Input: part model. Units: mm. Frame: model coordinates. A direction names the side the tool comes from. Give positions to 0.01 mm unless a question says otherwise; leave off trailing zeros. Loops run counter-clockwise (first coordinate to the right, second up) from the corner with the lowest first, then second, coordinate; pieces in that order, holes last. Notation, with made-up numbers: (44.5, 58) -> (52.5, 58) arc R17 cw to (52.5, 69) -> close; hole circle Ø9 at (71.5, 41). An arc over 180 degrees is marked (long way). Answer as a JSON object with one key per item and string values. Group by question number.
```python
from build123d import *

# Parameters (mm, degrees)
BOSS_EXTRUDE1_DEPTH = 6.35
CHAMFER1_SIZE       = 0.79375
CHAMFER2_SIZE       = 1.5875


with BuildPart() as part:
    # Sketch1 → Boss-Extrude1 (new body)
    with BuildSketch(Plane.XY):
        with BuildLine():
            Line((134.621545702, -67.612541882), (134.621545702, -60.810273898))
            ThreePointArc((134.621545702, -60.810273898), (134.621545702, -59.687741882), (133.499013687, -59.687741882))
            Line((133.499013687, -59.687741882), (102.049077718, -59.687741882))
            ThreePointArc((102.049077718, -59.687741882), (100.926545702, -59.687741882), (100.926545702, -60.810273898))
            Line((100.926545702, -60.810273898), (100.926545702, -67.612541882))
            Line((100.926545702, -67.612541882), (95.926545702, -67.612541882))
            Line((95.926545702, -67.612541882), (95.926545702, -60.810273898))
            ThreePointArc((95.926545702, -60.810273898), (95.926545702, -59.687741882), (94.804013687, -59.687741882))
            Line((94.804013687, -59.687741882), (-87.460922281, -59.687741882))
            ThreePointArc((-87.460922281, -59.687741882), (-88.583454296, -59.687741882), (-88.583454296, -60.810273898))
            Line((-88.583454296, -60.810273898), (-88.583454296, -67.612541882))
            Line((-88.583454296, -67.612541882), (-93.583454296, -67.612541882))
            Line((-93.583454296, -67.612541882), (-93.583454296, -60.810273898))
            ThreePointArc((-93.583454296, -60.810273898), (-93.583454296, -59.687741882), (-94.705986312, -59.687741882))
            Line((-94.705986312, -59.687741882), (-126.155922281, -59.687741882))
            ThreePointArc((-126.155922281, -59.687741882), (-127.278454296, -59.687741882), (-127.278454296, -60.810273898))
            Line((-127.278454296, -60.810273898), (-127.278454296, -67.612541882))
            Line((-127.278454296, -67.612541882), (-131.507694323, -67.612541882))
            Line((-131.507694323, -67.612541882), (-131.507694323, -62.385073898))
            ThreePointArc((-131.507694323, -62.385073898), (-131.507694323, -61.262541882), (-132.630226338, -61.262541882))
            Line((-132.630226338, -61.262541882), (-133.628454296, -61.262541882))
            Line((-133.628454296, -61.262541882), (-133.628454296, -60.810273898))
            ThreePointArc((-133.628454296, -60.810273898), (-133.628454296, -59.687741882), (-134.750986312, -59.687741882))
            Line((-134.750986312, -59.687741882), (-139.978454296, -59.687741882))
            Line((-139.978454296, -59.687741882), (-139.978454296, -58.735073898))
            ThreePointArc((-139.978454296, -58.735073898), (-139.978454296, -57.612541882), (-141.100986312, -57.612541882))
            Line((-141.100986312, -57.612541882), (-146.328454296, -57.612541882))
            Line((-146.328454296, -57.612541882), (-146.328454296, -47.612541882))
            Line((-146.328454296, -47.612541882), (-141.100986312, -47.612541882))
            ThreePointArc((-141.100986312, -47.612541882), (-139.978454296, -47.612541882), (-139.978454296, -46.490009867))
            Line((-139.978454296, -46.490009867), (-139.978454296, -38.735073898))
            ThreePointArc((-139.978454296, -38.735073898), (-139.978454296, -37.612541882), (-141.100986312, -37.612541882))
            Line((-141.100986312, -37.612541882), (-146.328454296, -37.612541882))
            Line((-146.328454296, -37.612541882), (-146.328454296, -27.612541882))
            Line((-146.328454296, -27.612541882), (-141.100986312, -27.612541882))
            ThreePointArc((-141.100986312, -27.612541882), (-139.978454296, -27.612541882), (-139.978454296, -26.490009867))
            Line((-139.978454296, -26.490009867), (-139.978454296, -20.787541882))
            Line((-139.978454296, -20.787541882), (-136.575986312, -20.787541882))
            ThreePointArc((-136.575986312, -20.787541882), (-135.453454296, -20.787541882), (-135.453454296, -19.665009867))
            Line((-135.453454296, -19.665009867), (-135.453454296, -17.612541882))
            Line((-135.453454296, -17.612541882), (-125.453454296, -17.612541882))
            Line((-125.453454296, -17.612541882), (-125.453454296, -19.665009867))
            ThreePointArc((-125.453454296, -19.665009867), (-125.453454296, -20.787541882), (-124.330922281, -20.787541882))
            Line((-124.330922281, -20.787541882), (-105.521454296, -20.787541882))
            Line((-105.521454296, -20.787541882), (-105.521454296, -29.665009867))
            ThreePointArc((-105.521454296, -29.665009867), (-105.521454296, -30.787541882), (-104.398922281, -30.787541882))
            Line((-104.398922281, -30.787541882), (-101.643986312, -30.787541882))
            ThreePointArc((-101.643986312, -30.787541882), (-100.521454296, -30.787541882), (-100.521454296, -29.665009867))
            Line((-100.521454296, -29.665009867), (-100.521454296, -20.787541882))
            Line((-100.521454296, -20.787541882), (-81.711986312, -20.787541882))
            ThreePointArc((-81.711986312, -20.787541882), (-80.589454296, -20.787541882), (-80.589454296, -19.665009867))
            Line((-80.589454296, -19.665009867), (-80.589454296, -17.612541882))
            Line((-80.589454296, -17.612541882), (-70.589454296, -17.612541882))
            Line((-70.589454296, -17.612541882), (-70.589454296, -23.005209867))
            ThreePointArc((-70.589454296, -23.005209867), (-70.589454296, -24.127741882), (-69.466922281, -24.127741882))
            Line((-69.466922281, -24.127741882), (76.810013687, -24.127741882))
            ThreePointArc((76.810013687, -24.127741882), (77.932545702, -24.127741882), (77.932545702, -23.005209867))
            Line((77.932545702, -23.005209867), (77.932545702, -17.612541882))
            Line((77.932545702, -17.612541882), (87.932545702, -17.612541882))
            Line((87.932545702, -17.612541882), (87.932545702, -19.665009867))
            ThreePointArc((87.932545702, -19.665009867), (87.932545702, -20.787541882), (89.055077718, -20.787541882))
            Line((89.055077718, -20.787541882), (131.674013687, -20.787541882))
            ThreePointArc((131.674013687, -20.787541882), (132.796545702, -20.787541882), (132.796545702, -19.665009867))
            Line((132.796545702, -19.665009867), (132.796545702, -17.612541882))
            Line((132.796545702, -17.612541882), (142.796545702, -17.612541882))
            Line((142.796545702, -17.612541882), (142.796545702, -19.665009867))
            ThreePointArc((142.796545702, -19.665009867), (142.796545702, -20.787541882), (143.919077718, -20.787541882))
            Line((143.919077718, -20.787541882), (147.321545702, -20.787541882))
            Line((147.321545702, -20.787541882), (147.321545702, -26.490009867))
            ThreePointArc((147.321545702, -26.490009867), (147.321545702, -27.612541882), (148.444077718, -27.612541882))
            Line((148.444077718, -27.612541882), (153.671545702, -27.612541882))
            Line((153.671545702, -27.612541882), (153.671545702, -37.612541882))
            Line((153.671545702, -37.612541882), (148.444077718, -37.612541882))
            ThreePointArc((148.444077718, -37.612541882), (147.321545702, -37.612541882), (147.321545702, -38.735073898))
            Line((147.321545702, -38.735073898), (147.321545702, -46.490009867))
            ThreePointArc((147.321545702, -46.490009867), (147.321545702, -47.612541882), (148.444077718, -47.612541882))
            Line((148.444077718, -47.612541882), (153.671545702, -47.612541882))
            Line((153.671545702, -47.612541882), (153.671545702, -57.612541882))
            Line((153.671545702, -57.612541882), (148.444077718, -57.612541882))
            ThreePointArc((148.444077718, -57.612541882), (147.321545702, -57.612541882), (147.321545702, -58.735073898))
            Line((147.321545702, -58.735073898), (147.321545702, -59.687741882))
            Line((147.321545702, -59.687741882), (142.094077718, -59.687741882))
            ThreePointArc((142.094077718, -59.687741882), (140.971545702, -59.687741882), (140.971545702, -60.810273898))
            Line((140.971545702, -60.810273898), (140.971545702, -61.262541882))
            Line((140.971545702, -61.262541882), (140.071500685, -61.262541882))
            ThreePointArc((140.071500685, -61.262541882), (138.948968669, -61.262541882), (138.948968669, -62.385073898))
            Line((138.948968669, -62.385073898), (138.948968669, -67.612541882))
            Line((138.948968669, -67.612541882), (134.621545702, -67.612541882))
        make_face()
    extrude(amount=BOSS_EXTRUDE1_DEPTH)

    # Chamfer1
    chamfer1_edges = [part.edges().sort_by_distance(p)[0] for p in [
        (100.926545702, -67.612541882, 3.175),
        (95.926545702, -67.612541882, 3.175),
        (-88.583454296, -67.612541882, 3.175),
        (-93.583454296, -67.612541882, 3.175),
        (-127.278454296, -67.612541882, 3.175),
        (-131.507694323, -67.612541882, 3.175),
        (-135.453454296, -17.612541882, 3.175),
        (-125.453454296, -17.612541882, 3.175),
        (-80.589454296, -17.612541882, 3.175),
        (-70.589454296, -17.612541882, 3.175),
        (77.932545702, -17.612541882, 3.175),
        (87.932545702, -17.612541882, 3.175),
        (132.796545702, -17.612541882, 3.175),
        (142.796545702, -17.612541882, 3.175),
        (138.948968669, -67.612541882, 3.175),
        (134.621545702, -67.612541882, 3.175),
    ]]
    chamfer(chamfer1_edges, length=CHAMFER1_SIZE)

    # Chamfer2
    chamfer2_edges = [part.edges().sort_by_distance(p)[0] for p in [
        (-146.328454296, -57.612541882, 3.175),
        (-146.328454296, -47.612541882, 3.175),
        (-146.328454296, -37.612541882, 3.175),
        (-146.328454296, -27.612541882, 3.175),
        (153.671545702, -27.612541882, 3.175),
        (153.671545702, -37.612541882, 3.175),
        (153.671545702, -47.612541882, 3.175),
        (153.671545702, -57.612541882, 3.175),
    ]]
    chamfer(chamfer2_edges, length=CHAMFER2_SIZE)


solid = part.part
```
Q1. Section B-B on x = 29. Return the cut outline in (y, z).
Q2. Pull-direction query (Y, two-part tool) for faces 1 (the face through (147.322, -43, 3)), 2 (the face through (95.927, -64, 3)), 3 (the face through (-115, -20.788, 3)); classes: +Y half, -Y half, draft (parallel to the pull), parting line (faces both ways), or undercut.
Q3. Section A-A on x = 120. Return the cut outline in (y, z).
Q4. Pin query (flat end, axial travel): pin 1 Ø0.6 at (y, z) = (-19, 3) entering from -X; pin 2 Ø3 at (y, z) = (-64.5, 2.5) entering from +X; pin 3 Ø0.8 at (x, z) = (-133.5, 2.5) entering from -Y. Return the tip coordinate at first contact, or that it passes through.
Q5. Ray query, probe 1 along X at (y, z) = (-63.5, 1); probe 2 along X at (y, z) = (-60.5, 4); probe 3 along X at (y, z) = (-24.5, 4.5). Return the intervals inside material, ascending.
Q6. Set-up query: faces 4 (the face through (-137, -59.688, 3)), 5 (the face through (110, -20.788, 3)), 6 (the face through (-139.978, -24, 3)), 7 (the face through (-93.583, -64, 3)). Return all of +Z, -Z, +X, -X, +Y, -Y with unobstructed straight access to the full face (end or side cutting, diameter ignored); none if empty.
Numbers:
{
 "1": {"outline": "(-59.69, 0) -> (-24.13, 0) -> (-24.13, 6.35) -> (-59.69, 6.35) -> close"},
 "2": {"face 1": "undercut", "face 2": "draft", "face 3": "+Y half"},
 "3": {"outline": "(-59.69, 0) -> (-20.79, 0) -> (-20.79, 6.35) -> (-59.69, 6.35) -> close"},
 "4": {"pin 1": "stops at x = -135.45", "pin 2": "stops at x = 138.95", "pin 3": "stops at y = -61.26"},
 "5": {"probe 1": "x = -131.51 to -127.28, -93.58 to -88.58, 95.93 to 100.93, 134.62 to 138.95", "probe 2": "x = -133.44 to -127.47, -93.39 to -88.78, 96.12 to 100.73, 134.81 to 140.78", "probe 3": "x = -139.98 to -105.52, -100.52 to 147.32"},
 "6": {"face 4": "+Z, -Z, -X, -Y", "face 5": "+Z, -Z, +Y", "face 6": "+Z, -Z, -X, +Y", "face 7": "+Z, -Z, -Y"}
}
